For this review, use the dimensioned drawing (mm, ordinates from the lowest corner) and the shaded views. Give positions to 0.01 mm unless a question says otherwise; leave off trailing zeros. Order: outer loops, then holes, each group sorted by start corner. A loop starts at its lowest first (then second) coordinate and runs counter-clockwise, first axis right, second up. Notation, with made-up numbers: (-8, 44.5) - (32, 44.5) arc R16 cw to (32, 73.5) - close; hole circle Ø11 at (51, -7). An arc over 180 degrees is marked (long way). One line per item, written item: value.
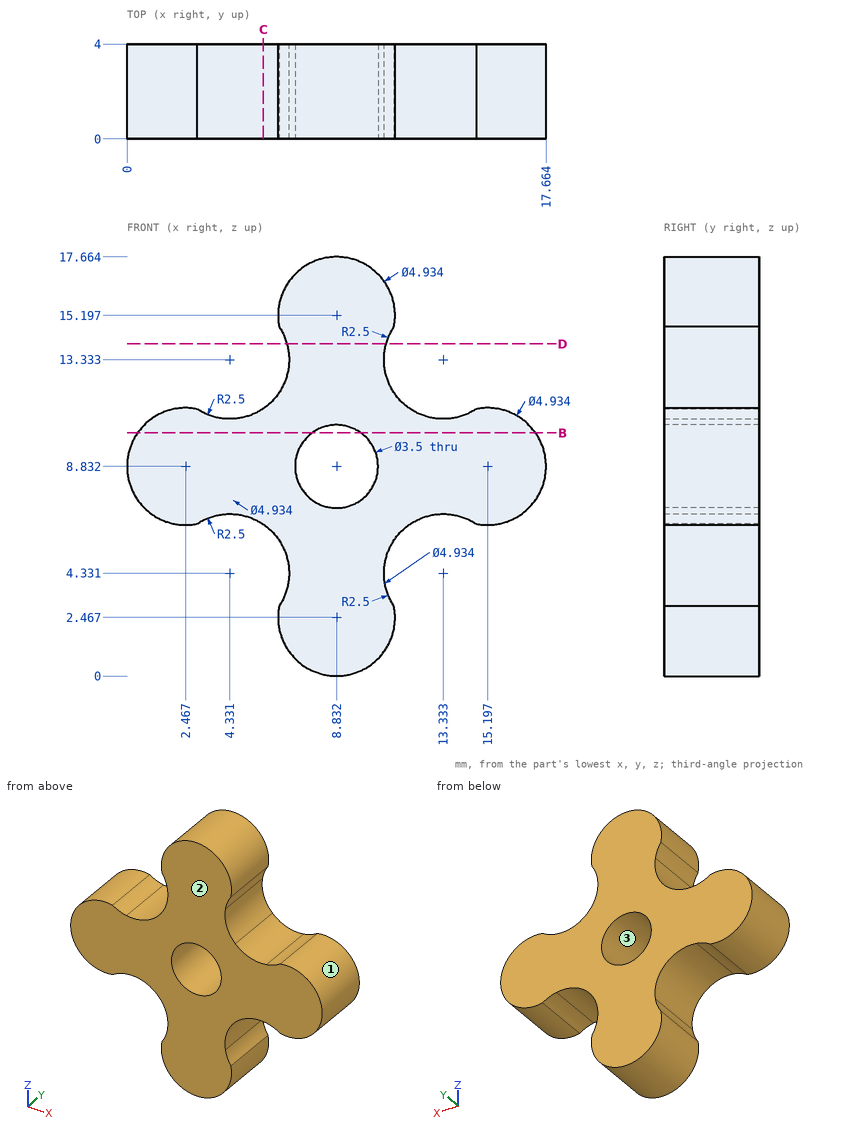
(1) Draft analysis for pull direction Z (two halves, no side actions). For the marked faces 1, 2 and 3, state which applies: pulls with the +Z half, pulls with the -Z half, needs draft (parallel to the pull), parting line crosses it, or undercut.
Answers below:
face 1: parting line crosses it
face 2: needs draft
face 3: undercut
(2) For P1, Ø2, axis at y = 0.5, z = 10.5, coming from the -X side; P2, Ø1.5, axis at y = 3, z = 15, coming from the -X side (3 decimals); P3, Ø1, axis at x = 15, y = 2, coming from the +Z side, all flat-tipped, find the tip position at first contact; note any pin that passes through.
Answers below:
P1: stops at x = 0.09
P2: stops at x = 6.365
P3: stops at z = 11.3
(3) Take a section at D-D (z = 14). Write out the cut boundary in (x, y).
Answers below:
outline: (6.74, 0) - (10.92, 0) - (10.92, 4) - (6.74, 4) - close
(4) Wall thickness on line 1 (X direction, y = 1.15, z = 8.75); line 2 (X direction, y = 3.4, z = 2) (1 decimal); line 3 (X direction, y = 1.6, z = 4.5) (1 decimal): over which ranges is each line inside the solid? List them lowest first. Write a range as from..to.
Answers below:
line 1: x = 0..7.08, 10.58..17.66
line 2: x = 6.4..11.3
line 3: x = 6.8..10.8
(5) Take a section at C-C (x = 5.75). Write out the cut boundary in (y, z).
Answers below:
outline: (0, 6.39) - (4, 6.39) - (4, 11.27) - (0, 11.27) - close
(6) Take a section at B-B (z = 10.25). Write out the cut boundary in (x, y).
Answers below:
outline: (0.45, 0) - (7.81, 0) - (7.81, 4) - (0.45, 4) - close; (9.86, 0) - (17.22, 0) - (17.22, 4) - (9.86, 4) - close
